Source: three-view drawing plus pictorial views. Frame: mm from the lowest corner of the part. A direction names the side the tool comes from. Coordinates: 2 decimals unless noted, no trailing zeros. Loops run counter-clockwise (first coordinate to the right, second up) from the corner with the lowest first, then second, coordinate; pieces in that order, holes last. Notation, with made-up numbers: M -32,42 L 23,42 A17 ccw 23,59 Z; hole C -39,40 d6. An arc over 180 degrees is marked long. Use a Markdown table: item, result. Add a question column.
1. Section C-C on z = 37.5. Output: boundary loops of the cut face in (x, y) (1 decimal).
2. Section D-D on y = 70. Output: boundary loops of the cut face in (x, z) (1 decimal), then the cut area to 3 significant figures.
3. Pin query (flat end, axial travel): pin 1 (6 mm diameter, centred on x = 16, y = 18.5, fed in from -Z) (1 decimal); pin 2 (4 mm diameter, centred on x = 16, y = 43, fed in from -Z) (1 decimal); pin 3 (5 mm diameter, centred on x = 14, z = 29.5, fed in from -Y) (1 decimal). Return the tip coordinate at first contact, or that it passes through.
4. Section A-A on y = 23. Output: boundary loops of the cut face in (x, z) (1 decimal).
5. Section B-B on x = 6. Output: boundary loops of the cut face in (y, z) (1 decimal), then the cut area to 3 significant figures.
6. Line query: L1, parallel to Y at x = 1, z = 25 (1 decimal); L2, parallel to Y at x = 15.75, z = 53 (1 decimal); L3, parallel to Y at x = 13.25, z = 37 (1 decimal). Output: solid intervals per line, ascending. Write a range as [from, to].
7. Draft query along Z for the marked faces 1, 2 and 3. Return one class per face: +Z half, -Z half, draft (parallel to the pull), parting line (faces both ways), or undercut.
8. Set-up query: the marked faces 4, 5 and 6. Return all of +Z, -Z, +X, -X, +Y, -Y with unobstructed straight access to the full face (end or side cutting, diameter ignored); none if empty.
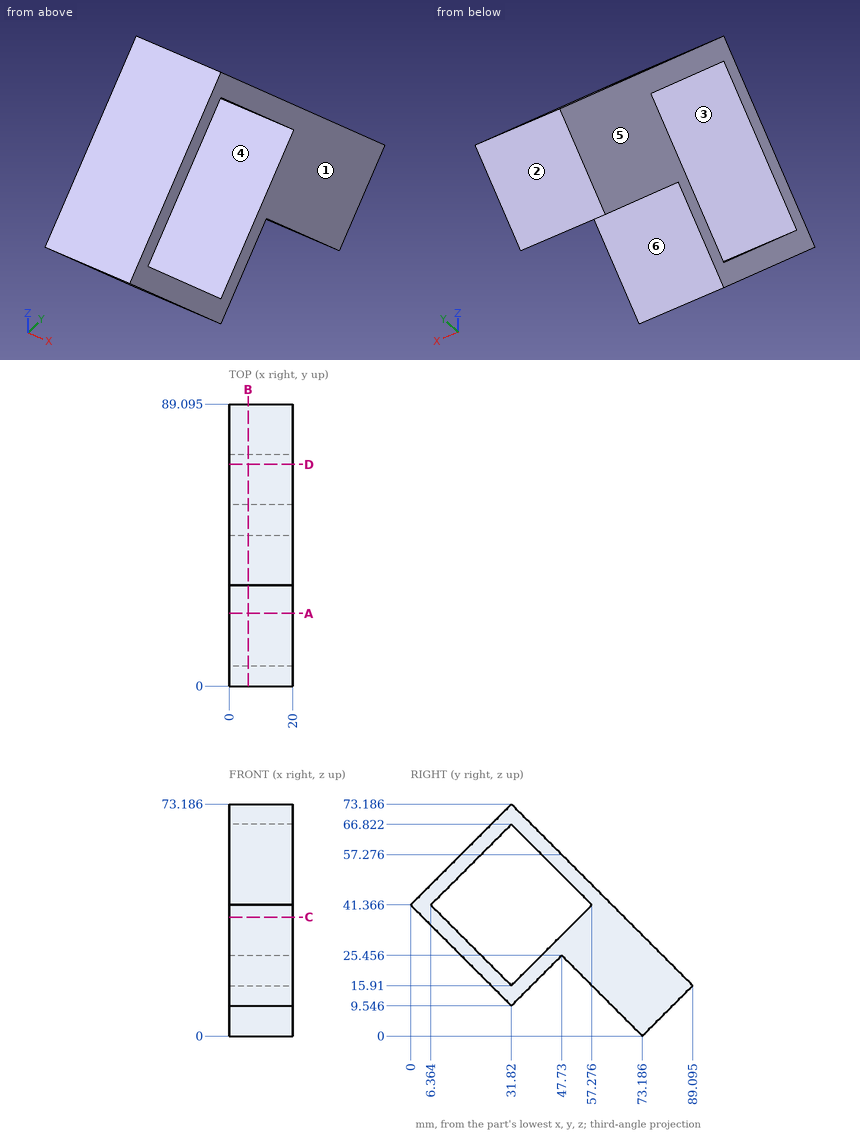
Answers below:
| question | item | result |
|---|---|---|
| 1 | outline | M 0,3.9 L 20,3.9 L 20,10.2 L 0,10.2 Z; M 0,53.4 L 20,53.4 L 20,67.5 L 0,67.5 Z |
| 2 | outline | M 0,3.2 L 20,3.2 L 20,35 L 0,35 Z |
| 2 | area | 636 mm² |
| 3 | pin 1 | stops at z = 19.9 |
| 3 | pin 2 | stops at z = 18.7 |
| 3 | pin 3 | stops at y = 9.4 |
| 4 | outline | M 0,18.4 L 20,18.4 L 20,24.7 L 0,24.7 Z; M 0,58 L 20,58 L 20,64.4 L 0,64.4 Z |
| 5 | outline | M 0,41.4 L 31.8,9.5 L 47.7,25.5 L 73.2,0 L 89.1,15.9 L 31.8,73.2 Z; hole M 6.4,41.4 L 31.8,15.9 L 57.3,41.4 L 31.8,66.8 Z |
| 5 | area | 1,540 mm² |
| 6 | L1 | y = [16.4, 22.7], [40.9, 47.3], [48.2, 80] |
| 6 | L2 | y = [11.6, 18], [45.6, 52] |
| 6 | L3 | y = [4.4, 10.7], [52.9, 68] |
| 7 | face 1 | draft |
| 7 | face 2 | -Z half |
| 7 | face 3 | undercut |
| 8 | face 4 | +X, -X |
| 8 | face 5 | +Z, -Z, -X, +Y, -Y |
| 8 | face 6 | -Z, +X, -X |
